from build123d import *

# Parameters (mm, degrees)
SKETCH1_R           = 1
SKETCH1_R_2         = 1.5
SKETCH1_R_3         = 2
SKETCH1_W           = 23
SKETCH1_H           = 12
BOSS_EXTRUDE1_DEPTH = 2.5
FILLET1_R           = 3.5


with BuildPart() as part:
    # Sketch1 → Boss-Extrude1 (new body)
    with BuildSketch(Plane.XY):
        with BuildLine():
            Line((-17.5, 9), (-17.5, -19))
            Line((-17.5, -19), (17.5, -19))
            Line((17.5, -19), (17.5, 9))
            ThreePointArc((17.5, 9), (0, 26), (-17.5, 9))
        make_face()
        with Locations((-14, 0)):
            Circle(SKETCH1_R, mode=Mode.SUBTRACT)
        with Locations((-14, -10)):
            Circle(SKETCH1_R_2, mode=Mode.SUBTRACT)
        with Locations((-8.5, 16)):
            Circle(SKETCH1_R_3, mode=Mode.SUBTRACT)
        with Locations((14, -10)):
            Circle(SKETCH1_R_2, mode=Mode.SUBTRACT)
        with Locations((14, 0)):
            Circle(SKETCH1_R, mode=Mode.SUBTRACT)
        with Locations((8.5, 16)):
            Circle(SKETCH1_R_3, mode=Mode.SUBTRACT)
        Rectangle(SKETCH1_W, SKETCH1_H, mode=Mode.SUBTRACT)
        with BuildLine():
            Line((-6.2, -13.5), (6.2, -13.5))
            ThreePointArc((6.2, -13.5), (7.7, -15), (6.2, -16.5))
            Line((6.2, -16.5), (-6.2, -16.5))
            ThreePointArc((-6.2, -16.5), (-7.7, -15), (-6.2, -13.5))
        make_face(mode=Mode.SUBTRACT)
    extrude(amount=BOSS_EXTRUDE1_DEPTH)

    # Fillet1
    fillet1_edges = [part.edges().sort_by_distance(p)[0] for p in [
        (17.5, -19, 1.25),
        (-17.5, -19, 1.25),
    ]]
    fillet(fillet1_edges, radius=FILLET1_R)


solid = part.part
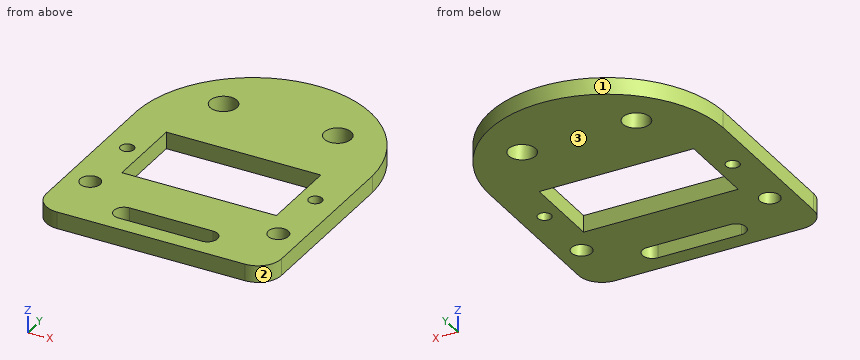
Input: part model. Units: mm. Frame: model coordinates. Face numbers are marked on the shaded views. Coordinates: 2 decimals unless noted, no trailing zeros. Loops run counter-clockwise (first coordinate to the right, second up) from the corner with the lowest first, then second, coordinate; pieces in that order, holes last. Notation, with made-up numbers: (-2, -29) -> (50, -29) arc R26 cw to (50, 0) -> close; hole circle Ø8 at (32, -38.75). An arc over 180 degrees is marked (long way). Write item = value, one per line. Start each with the question number.
Item 1: Material intervals for line 1 (X direction, y = 4.5, z = 1.8); line 2 (Y direction, x = -8.5, z = 0.9); line 3 (Y direction, x = -3.5, z = 0.6), sorted ascending.
Item 2: Cut plane B-B, the plane z = 1.45. Count the separate pieces of the cut face and the enclosed holes in it, plus the area to 3 significant figures.
Item 3: Cut plane D-D, the plane y = -10. Return loops of the section in (x, z), plus the area to 3 significant figures.
Item 4: Cut plane A-A, the plane y = 2.5. Return loops of the section in (x, z).
Item 5: Cut plane C-C, the plane x = 9.5. Return loops of the section in (y, z), plus the area to 3 significant figures.
Item 6: Mould query, pull axis Y, two halves, no side actions, for the marked faces 1, 2 and 3. Classes: pulls with the +Y half, pulls with the -Y half, needs draft (parallel to the pull), parting line crosses it, or undercut.
Ans:
q1.line_1 = -17.5 to -11.5, 11.5 to 17.5
q1.line_2 = -19 to -6, 6 to 14, 18 to 23.8
q1.line_3 = -19 to -16.5, -13.5 to -6, 6 to 25.65
q2.separate_pieces = 1
q2.enclosed_holes = 8
q2.area = 1,070 mm²
q3.outline = (-17.5, 0) -> (-15.5, 0) -> (-15.5, 2.5) -> (-17.5, 2.5) -> close; (-12.5, 0) -> (12.5, 0) -> (12.5, 2.5) -> (-12.5, 2.5) -> close; (15.5, 0) -> (17.5, 0) -> (17.5, 2.5) -> (15.5, 2.5) -> close
q3.area = 72.5 mm²
q4.outline = (-17.5, 0) -> (-11.5, 0) -> (-11.5, 2.5) -> (-17.5, 2.5) -> close; (11.5, 0) -> (17.5, 0) -> (17.5, 2.5) -> (11.5, 2.5) -> close
q5.outline = (-19, 0) -> (-6, 0) -> (-6, 2.5) -> (-19, 2.5) -> close; (6, 0) -> (14.27, 0) -> (14.27, 2.5) -> (6, 2.5) -> close; (17.73, 0) -> (23.2, 0) -> (23.2, 2.5) -> (17.73, 2.5) -> close
q5.area = 66.8 mm²
q6.face_1 = pulls with the +Y half
q6.face_2 = pulls with the -Y half
q6.face_3 = needs draft
